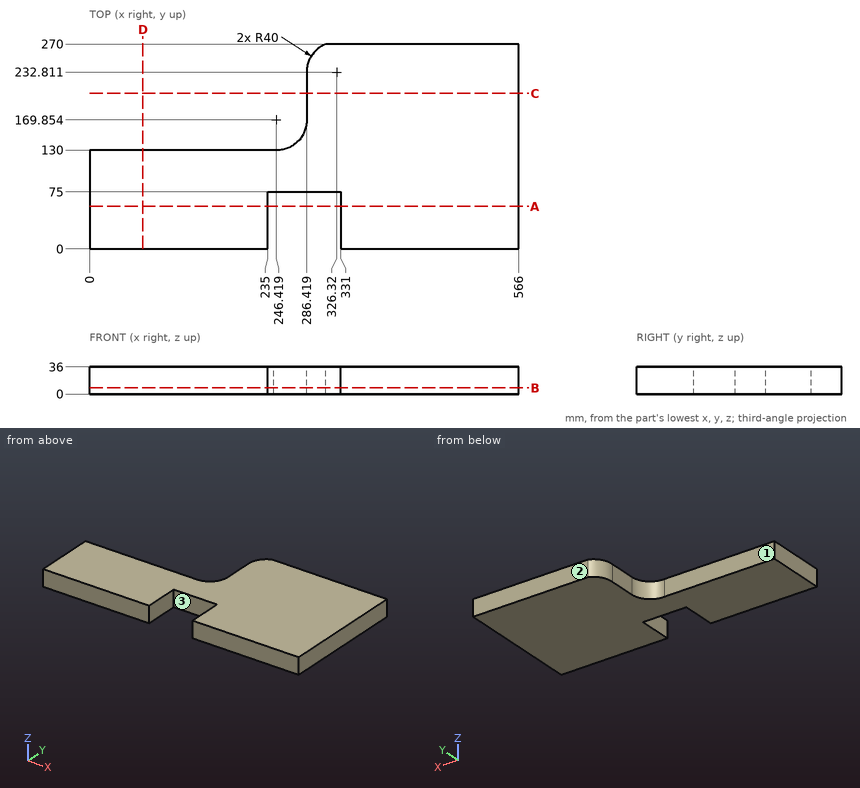
Here's the drawing with two shaded views (mm, measured from the low corner). I have some questions. A direction names the side the tool comes from. Round coordinates to 2 decimals unless told otherwise and drop trailing zeros. Write each loop counter-clockwise with the first axis right and the second up, starting at its lowest first coordinate (ties: lowest second). Pieces come first, ordered by that corner, then holes. Notation, with made-up numbers: M -14.75,14 L 42.25,14 A27 cw 42.25,50 Z; hole C -32.5,-36 d9. An arc over 180 degrees is marked long. Answer in a Markdown table with one row per item. Add a question column.
Q1. Imagine slicing it at A-A (y = 56). Please give me the cut outline in (x, z), then the cut area to 3 significant figures.
Q2. Will these pins go through, and if not, where does the flat tip stop? pin 1 Ø4 at (x, z) = (208, 12) entering from +Y; pin 2 Ø2 at (x, z) = (235, 13) entering from -Y; pin 3 Ø1.5 at (y, z) = (182.5, 23) entering from -X; pin 4 Ø18 at (x, z) = (303.5, 11.5) entering from -Y.
Q3. Imagine slicing it at D-D (x = 70.5). Please give me the cut outline in (y, z), then the cut area to 3 significant figures.
Q4. If I drill on line 1 (X direction, y = 52, z = 13); line 2 (X direction, y = 220, z = 20); line 3 (Y direction, x = 99, z = 5), over which ranges is the centre line in solid material (lowest first)? Write a range as from..to.
Q5. Imagine slicing it at C-C (y = 205). Please give me the cut outline in (x, z).
Q6. Imagine slicing it at B-B (z = 8). Please give me the cut outline in (x, y), then the cut area to 3 significant figures.
Q7. On a 3-axis mill with a long thin cutter (end or side, diameter ignored), from which of +Z, -Z, +X, -X, +Y, -Y can I reach the whole of each face in a straight line? I mean the marked faces 1, 2 and 3. Say none if no direction works.
Values:
| question | item | result |
|---|---|---|
| 1 | outline | M 0,0 L 235,0 L 235,36 L 0,36 Z; M 331,0 L 566,0 L 566,36 L 331,36 Z |
| 1 | area | 16,900 mm^2 |
| 2 | pin 1 | y = 130 |
| 2 | pin 2 | y = 0 |
| 2 | pin 3 | x = 286.42 |
| 2 | pin 4 | y = 75 |
| 3 | outline | M 0,0 L 130,0 L 130,36 L 0,36 Z |
| 3 | area | 4,680 mm^2 |
| 4 | line 1 | 0..235, 331..566 |
| 4 | line 2 | 286.42..566 |
| 4 | line 3 | 0..130 |
| 5 | outline | M 286.42,0 L 566,0 L 566,36 L 286.42,36 Z |
| 6 | outline | M 0,0 L 235,0 L 235,75 L 331,75 L 331,0 L 566,0 L 566,270 L 311.59,270 A40 ccw 286.42,230 L 286.42,170 A40 cw 243,130 L 0,130 Z |
| 6 | area | 106,000 mm^2 |
| 7 | face 1 | +Z, -Z, -X, +Y |
| 7 | face 2 | +Z, -Z, +X, -X, +Y |
| 7 | face 3 | +Z, -Z, -Y |
